Verification items for the finished model (mm, model axes). A direction names the side the tool comes from. Coordinates: 2 decimals unless noted, no trailing zeros. Loops run counter-clockwise (first coordinate to the right, second up) from the corner with the lowest first, then second, coordinate; pieces in that order, holes last. Notation, with made-up numbers: M 58,65.5 L 69,65.5 A21 ccw 69,75.5 Z; hole C 15.25,15 d3. An arc over 180 degrees is marked long. Write item = value, one per line. Start each with the question number.
```python
from build123d import *

# Parameters (mm, degrees)
BOSS_EXTRUDE1_DEPTH = 6.35
SKETCH2_R           = 1.1303
CUT_EXTRUDE1_DEPTH  = 12.7
FILLET1_R           = 2.54


with BuildPart() as part:
    # Sketch1 → Boss-Extrude1 (new body)
    with BuildSketch(Plane(origin=(0, 0, 0), x_dir=(1, 0, 0), z_dir=(0, 1, 0))):
        with BuildLine():
            Line((-21.5138, -15.875), (-9.729950234, -15.875))
            Line((-9.729950234, -15.875), (-9.729950234, -15.176835913))
            ThreePointArc((-9.729950234, -15.176835913), (-5.035098569, -13.262737362), (0, -12.668441286))
            ThreePointArc((0, -12.668441286), (5.035098569, -13.262737362), (9.729950234, -15.176835913))
            Line((9.729950234, -15.176835913), (9.729950234, -15.875))
            Line((9.729950234, -15.875), (21.5138, -15.875))
            Line((21.5138, -15.875), (21.5138, -6.223))
            Line((21.5138, -6.223), (27.8638, -6.223))
            Line((27.8638, -6.223), (27.8638, 6.1722))
            Line((27.8638, 6.1722), (21.5138, 6.1722))
            Line((21.5138, 6.1722), (21.5138, 13.335))
            Line((21.5138, 13.335), (-21.5138, 13.335))
            Line((-21.5138, 13.335), (-21.5138, 6.1722))
            Line((-21.5138, 6.1722), (-27.8638, 6.1722))
            Line((-27.8638, 6.1722), (-27.8638, -6.223))
            Line((-27.8638, -6.223), (-21.5138, -6.223))
            Line((-21.5138, -6.223), (-21.5138, -15.875))
        make_face()
    extrude(amount=BOSS_EXTRUDE1_DEPTH)

    # Sketch2 → Cut-Extrude1 (cut)
    with BuildSketch(Plane.ZY.offset(21.5138)):
        with Locations((-11.1125, 3.175)):
            Circle(SKETCH2_R)
        with Locations(Location((11.1125, 3.175, 0), (0, 0, 180))):
            Circle(SKETCH2_R)
    cut_extrude1 = extrude(amount=-CUT_EXTRUDE1_DEPTH, mode=Mode.SUBTRACT)

    # Mirror1: Cut-Extrude1 across plane
    add(cut_extrude1.mirror(Plane(origin=(0, 0, 0), x_dir=(0, 0, 1), z_dir=(1, 0, 0))), mode=Mode.SUBTRACT)

    # Fillet1
    # the kernel refuses this fillet: 2.54 mm, written as the material it takes off along each edge
    with BuildSketch(Plane(origin=(9.729950234, -4.372671145, 15.875), x_dir=(0, 0, -1), z_dir=(0, 1, 0))) as fillet1_piece_1:
        with BuildLine():
            CenterArc((2.54, -1.749068458), FILLET1_R, 136.479850512, 43.520149488)
            Line((0, -1.749068458), (-0.0508, -1.749068458))
            Line((-0.0508, -1.749068458), (-0.0508, 0))
            Line((-0.0508, 0), (0, 0.0508))
            ThreePointArc((0, 0.0508), (0.349082044, 0.0508), (0.661327369, 0.034981369))
            Line((0.661327369, 0.034981369), (0.698164087, 0))
        make_face()
    extrude(amount=15.095342289, mode=Mode.SUBTRACT)
    with BuildSketch(Plane(origin=(-9.729950234, -4.372671145, 15.875), x_dir=(-1, 0, 0), z_dir=(0, 1, 0))) as fillet1_piece_2:
        with BuildLine():
            CenterArc((1.749068458, -2.54), FILLET1_R, 90, 43.520149488)
            Line((0, -0.698164087), (-0.034981369, -0.661327369))
            ThreePointArc((-0.034981369, -0.661327369), (-0.0508, -0.349082044), (-0.0508, 0))
            Line((-0.0508, 0), (0, 0.0508))
            Line((0, 0.0508), (1.749068458, 0.0508))
            Line((1.749068458, 0.0508), (1.749068458, 0))
        make_face()
    extrude(amount=15.095342289, mode=Mode.SUBTRACT)


solid = part.part
```
Q1. Mould release check, pull along X, two halves, no side actions. Record for faces 5 (the face through (-25, 3, 6.223)), 6 (the face through (-21.514, 3.1, -9.8)), 7 (the face through (-5.1, 3.13, 13.28)): +X half, -X half, draft (parallel to the pull), parting line (faces both ways), or undercut.
Q2. Sectioned sample at B-B on x = -21. Count the separate pieces of the cut face and the enclosed holes in it, plus the area to 3 significant figures.
Q3. Scan lines: L1, parallel to Y at x = 9.5, z = 11; L2, parallel to X at y = 5, z = 8; L3, parallel to Z at x = -19.5, y = 2.25 (3 decimals). Record each from-to range of solid material in increasing order. Write a range as [from, to].
Q4. Sectioned sample at C-C on y = 5.75. Record the cut outline in (x, z) (3 decimals), plus the area to 3 significant figures.
Q5. Set-up check for faces 1 (the face through (-21.514, 4, 10)), 2 (the face through (25, 3, 6.223)), 3 (the face through (-10.55, 3.13, 15.7)), 4 (the face through (8.814, 3, 11)): record each of +Z, -Z, +X, -X, +Y, -Y from which the full face is reachable in a straight line by a thin tool's end or side.
Q6. Sectioned sample at A-A on z = 13.75. Record the cut outline in (x, y).
Q7. Gauge pin test, flat ends, axial feed: pin 1 (1.1 mm diameter, centred on y = 3, z = 11, fed in from -X); pin 2 (1 mm diameter, centred on y = 3.5, z = 10, fed in from +X); pin 3 (1.8 mm diameter, centred on y = 3.18, z = 11.11, fed in from +X); pin 4 (3 mm diameter, centred on x = -9, z = 12.5, fed in from -Y). Record the tip position at first contact, or that the pin passes through.
Q8. Sectioned sample at D-D on z = -7.5. Record the cut outline in (x, y), plus the area to 3 significant figures.
Solutions:
q1.face_5 = draft
q1.face_6 = -X half
q1.face_7 = undercut
q2.separate_pieces = 1
q2.enclosed_holes = 2
q2.area = 177 mm²
q3.L1 = [0, 2.05], [4.3, 6.35]
q3.L2 = [-21.51, 21.51]
q3.L3 = [-13.335, -11.762], [-10.463, 10.463], [11.762, 15.875]
q4.outline = M -27.864,-6.172 L -21.514,-6.172 L -21.514,-13.335 L 21.514,-13.335 L 21.514,-6.172 L 27.864,-6.172 L 27.864,6.223 L 21.514,6.223 L 21.514,15.875 L 11.479,15.875 A2.54 ccw 9.73,15.177 A18.86 cw 0,12.668 A18.86 cw -9.73,15.177 A2.54 ccw -11.479,15.875 L -21.514,15.875 L -21.514,6.223 L -27.864,6.223 Z
q4.area = 1,370 mm²
q5.face_1 = +Z, -X, +Y, -Y
q5.face_2 = +Z, +X, +Y, -Y
q5.face_3 = +Z, +Y, -Y
q5.face_4 = +X
q6.outline = M -21.51,0 L -6.63,0 L -6.63,6.35 L -21.51,6.35 Z; M 6.63,0 L 21.51,0 L 21.51,6.35 L 6.63,6.35 Z
q7.pin_1 = -8.81
q7.pin_2 = 21.51
q7.pin_3 = 8.81
q7.pin_4 = 0
q8.outline = M -21.51,0 L 21.51,0 L 21.51,6.35 L -21.51,6.35 Z
q8.area = 273 mm²
